from build123d import *

# Parameters (mm, degrees)
SKETCH1_W           = 49
SKETCH1_H           = 22
BOSS_EXTRUDE1_DEPTH = 3
BOSS_EXTRUDE2_DEPTH = 22
BOSS_EXTRUDE3_DEPTH = 3
CUT_EXTRUDE1_DEPTH  = 3


with BuildPart() as part:
    # Sketch1 → Boss-Extrude1 (new body)
    with BuildSketch(Plane(origin=(0, 0, 0), x_dir=(1, 0, 0), z_dir=(0, 1, 0))):
        with Locations((-24.5, 11)):
            Rectangle(SKETCH1_W, SKETCH1_H)
    extrude(amount=BOSS_EXTRUDE1_DEPTH)

    # Sketch2 → Boss-Extrude2 (add)
    with BuildSketch(Plane.XY):
        Polygon((0, 0), (0, -3.5), (4, -3.5), (4, 3), (0, 3), align=None)
    extrude(amount=-BOSS_EXTRUDE2_DEPTH)

    # Sketch3 → Boss-Extrude3 (add)
    with BuildSketch(Plane.XZ.offset(3.5)):
        Polygon((0, 0), (-60, 0), (-60, -22), (0, -22), (4, -22), (4, 0), align=None)
    extrude(amount=BOSS_EXTRUDE3_DEPTH)

    # Sketch4 → Cut-Extrude1 (cut)
    with BuildSketch(Plane.XZ.offset(6.5)):
        with BuildLine():
            Line((-56.05, -8.95), (-54, -8.95))
            ThreePointArc((-54, -8.95), (-51.95, -11), (-54, -13.05))
            Line((-54, -13.05), (-56.05, -13.05))
            ThreePointArc((-56.05, -13.05), (-58.1, -11), (-56.05, -8.95))
        make_face()
    extrude(amount=-CUT_EXTRUDE1_DEPTH, mode=Mode.SUBTRACT)


solid = part.part
Check sheet for the modelled part. Datum: model origin and axes. Units: mm. A direction names the side the tool comes from. Coordinates: 2 decimals unless noted, no trailing zeros. Write each loop counter-clockwise with the first axis right and the second up, starting at its lowest first coordinate (ties: lowest second). Pieces come first, ordered by that corner, then holes.
Item 1: Cross-section at D-D on y = -2.75. Record the boundary of the cut face in (x, z).
Numbers:
outline: (0, -22) - (4, -22) - (4, 0) - (0, 0) - close
Item 2: Cross-section at B-B on x = -20. Record the boundary of the cut face in (y, z).
Numbers:
outline: (-6.5, -22) - (-3.5, -22) - (-3.5, 0) - (-6.5, 0) - close; (0, -22) - (3, -22) - (3, 0) - (0, 0) - close
Item 3: Cross-section at C-C on z = -6.25. Record the boundary of the cut face in (x, y).
Numbers:
outline: (-60, -6.5) - (4, -6.5) - (4, 3) - (-49, 3) - (-49, 0) - (0, 0) - (0, -3.5) - (-60, -3.5) - close
Item 4: Scan lines: probe 1 along Y at (x, z) = (-43.5, -6.75); probe 2 along X at (y, z) = (-0.5, -6.75); probe 3 along X at (y, z) = (1.5, -19.5). Record each from-to range of solid material in increasing order.
Numbers:
probe 1: y = -6.5 to -3.5, 0 to 3
probe 2: x = 0 to 4
probe 3: x = -49 to 4
Item 5: Mould release check, pull along X, two halves, no side actions. Record for faces 4 (the face through (-58.1, -5, -11)), 5 (the face through (-28, -4, 0)), 6 (the face through (-49, 1, -11)): released by +X, released by -X, zero draft, split by the parting line, or undercut.
Numbers:
face 4: undercut
face 5: zero draft
face 6: released by -X
Item 6: Depth check by flat-ended pin: pin 1 Ø4 at (x, y) = (-32.5, -1.5) entering from -Z; pin 2 Ø1.5 at (y, z) = (2, -8.5) entering from -X; pin 3 Ø1.8 at (y, z) = (-1.5, -12) entering from -X. Enter the tip coordinate at first touch or a pass-through.
Numbers:
pin 1: stops at z = -22
pin 2: stops at x = -49
pin 3: stops at x = 0
Item 7: Cross-section at A-A on z = -11. Record the boundary of the cut face in (x, y), then the cut area to 3 significant figures.
Numbers:
outline: (-60, -6.5) - (-58.1, -6.5) - (-58.1, -3.5) - (-60, -3.5) - close; (-51.95, -6.5) - (4, -6.5) - (4, 3) - (-49, 3) - (-49, 0) - (0, 0) - (0, -3.5) - (-51.95, -3.5) - close
area: 347 mm2
Item 8: Access from +Z, -Z, +X, -X, +Y, -Y to the whole of each face (thin tool, end or side, straight path). Record for faces 1 (the face through (-28, -6.5, -11)), 2 (the face through (0, -2, -11)), 3 (the face through (-55, -5, -13.05)).
Numbers:
face 1: +Z, -Z, +X, -X, -Y
face 2: +Z, -Z, -X
face 3: +Y, -Y
